Geometry check sheet. Reference: the model listing, model coordinates, mm. Round coordinates to 2 decimals unless told otherwise and drop trailing zeros. Write each loop counter-clockwise with the first axis right and the second up, starting at its lowest first coordinate (ties: lowest second). Pieces come first, ordered by that corner, then holes. Notation, with made-up numbers: (84.25, 24.5) -> (125.25, 24.5) arc R13 ccw to (125.25, 41.5) -> close; hole circle Ø2 at (7.5, 7). An arc over 180 degrees is marked (long way). Return JSON: item names as keys, results as strings. Group by question number.
from build123d import *

# Parameters (mm, degrees)
SALIENTE_EXTRUIR1_DEPTH = 6
CROQUIS2_W              = 30
CROQUIS2_H              = 6
SALIENTE_EXTRUIR2_DEPTH = 6
CORTAR_EXTRUIR1_REACH   = 8
CROQUIS3_W              = 5.8
CROQUIS3_H              = 29.8
REDONDEO1_R             = 20
REDONDEO2_R             = 5


with BuildPart() as part:
    # Croquis1 → Saliente-Extruir1 (new body)
    with BuildSketch(Plane.XY):
        Polygon((-90, -40), (-34, 50), (306, 50), (306, 0), (0, 0), (0, -40), align=None)
    extrude(amount=SALIENTE_EXTRUIR1_DEPTH)

    # Croquis2 → Saliente-Extruir2 (add)
    with BuildSketch(Plane.XZ.offset(40)):
        with Locations((-75, 3)):
            Rectangle(CROQUIS2_W, CROQUIS2_H)
        with Locations((-15, 3)):
            Rectangle(CROQUIS2_W, CROQUIS2_H)
    extrude(amount=SALIENTE_EXTRUIR2_DEPTH)

    # Croquis3 → Cortar-Extruir1 (cut, up to next)
    with BuildSketch(Plane.XY.offset(6), mode=Mode.PRIVATE) as cortar_extruir1_sk1:
        with Locations((-2.9, 25)):
            Rectangle(CROQUIS3_W, CROQUIS3_H)
    cortar_extruir1_tool1 = extrude(cortar_extruir1_sk1.sketch, amount=-CORTAR_EXTRUIR1_REACH, mode=Mode.PRIVATE) & part.part
    add(cortar_extruir1_tool1.solids().sort_by_distance((-2.9, 25, 6))[0], mode=Mode.SUBTRACT)
    # Croquis3 → Cortar-Extruir1 (cut, up to next)
    with BuildSketch(Plane.XY.offset(6), mode=Mode.PRIVATE) as cortar_extruir1_sk2:
        with Locations((291.3, 25)):
            Rectangle(CROQUIS3_W, CROQUIS3_H)
    cortar_extruir1_tool2 = extrude(cortar_extruir1_sk2.sketch, amount=-CORTAR_EXTRUIR1_REACH, mode=Mode.PRIVATE) & part.part
    add(cortar_extruir1_tool2.solids().sort_by_distance((291.3, 25, 6))[0], mode=Mode.SUBTRACT)

    # Redondeo1
    redondeo1_edges = [part.edges().sort_by_distance(p)[0] for p in [
        (-34, 50, 3),
        (0, 0, 3),
    ]]
    fillet(redondeo1_edges, radius=REDONDEO1_R)

    # Redondeo2
    redondeo2_edges = [part.edges().sort_by_distance(p)[0] for p in [
        (306, 50, 3),
        (306, 0, 3),
    ]]
    fillet(redondeo2_edges, radius=REDONDEO2_R)


solid = part.part
1) Sectioned sample at B-B on y = 30. Enter the section's corners in (x, z), and give its area (3 significant figures).
2) Material ranges on probe 1 along X at (y, z) = (-42, 3.35); probe 2 along X at (y, z) = (39, 0.45); probe 3 along Y at (x, z) = (153, 4.9), recorded low to high. Write a range as [from, to].
3) Sectioned sample at D-D on y = -24. Enter the section's corners in (x, z), and give its area (3 significant figures).
4) Sectioned sample at A-A on z = 1.8. Enter the section's corners in (x, y), and give its area (4 significant figures).
5) Go/stop test with flat-tipped pins: P1, Ø1.5, axis at x = 69, y = 0, coming from the -Z side; P2, Ø3, axis at y = -36.5, z = 1.5, coming from the +X side; P3, Ø2, axis at y = 9, z = 4, coming from the -X side. Record where each tip stops, or that it passes through.
6) Sectioned sample at C-C on x = 249.5. Enter the section's corners in (y, z).
Evaluation:
{
 "1": {"outline": "(-46.44, 0) -> (-5.8, 0) -> (-5.8, 6) -> (-46.44, 6) -> close; (0, 0) -> (288.4, 0) -> (288.4, 6) -> (0, 6) -> close; (294.2, 0) -> (306, 0) -> (306, 6) -> (294.2, 6) -> close", "area": "2,050 mm2"},
 "2": {"probe 1": "x = [-90, -60], [-30, 0]", "probe 2": "x = [-40.84, -5.8], [0, 288.4], [294.2, 306]", "probe 3": "y = [0, 50]"},
 "3": {"outline": "(-80.04, 0) -> (0, 0) -> (0, 6) -> (-80.04, 6) -> close", "area": "480 mm2"},
 "4": {"outline": "(-90, -46) -> (-60, -46) -> (-60, -40) -> (-30, -40) -> (-30, -46) -> (0, -46) -> (0, -20) arc R20 cw to (20, 0) -> (301, 0) arc R5 ccw to (306, 5) -> (306, 45) arc R5 ccw to (301, 50) -> (-22.89, 50) arc R20 ccw to (-39.87, 40.57) -> (-90, -40) -> close; hole (-5.8, 10.1) -> (0, 10.1) -> (0, 39.9) -> (-5.8, 39.9) -> close; hole (288.4, 10.1) -> (294.2, 10.1) -> (294.2, 39.9) -> (288.4, 39.9) -> close", "area": "20,950 mm2"},
 "5": {"P1": "stops at z = 0", "P2": "stops at x = 0", "P3": "stops at x = -60.13"},
 "6": {"outline": "(0, 0) -> (50, 0) -> (50, 6) -> (0, 6) -> close"}
}
